Verification items for the finished model (mm, model axes). Round coordinates to 2 decimals unless told otherwise and drop trailing zeros. Order: outer loops, then holes, each group sorted by start corner. A loop starts at its lowest first (then second) coordinate and runs counter-clockwise, first axis right, second up. Notation, with made-up numbers: (45.25, -9.5) -> (66.25, -9.5) arc R32 cw to (66.25, 27.5) -> close; hole circle Ø10 at (18, 26). An arc over 180 degrees is marked (long way). Return JSON: item names as keys, results as strings. Group by question number.
Item 1: Scan lines: probe 1 along Y at (x, z) = (-41, 0.4); probe 2 along X at (y, z) = (-35, 0.4); probe 3 along Y at (x, z) = (-42.25, 0.15). Record each from-to range of solid material in increasing order. Write a range as from..to.
Item 2: Sectioned sample at B-B on x = -40. Record the cut outline in (y, z), plus the area to 3 significant figures.
Item 3: Sectioned sample at A-A on x = -47.25. Record the cut outline in (y, z).
Autodesk Fusion 360 part; units mm, degrees
sketch "Sketch1" plane through (0, 0, 0) normal (0, 0, 1) x (1, 0, 0)
  line L0 (-33, -71.5) -> (-33, -39.0517)
  spline S0 degree 3 poles (-33, -39.0517) (-33, -37.2602) (-33.4854, -35.4836) (-34.2537, -34.2725) (-34.9261, -33.2125) (-35.7722, -32.611) (-36.5563, -32.4575) (-37.1254, -32.346) (-37.6904, -32.44) (-38.2678, -32.7734) knots -1.570796 -1.570796 -1.570796 -1.570796 -0.801145 -0.801145 -0.801145 -0.12753 -0.12753 -0.12753 0.361367 0.361367 0.361367 0.361367
  line L1 (-38.2678, -32.7734) -> (-50, -39.547)
  line L2 (-50, -39.547) -> (-50, -71.5)
  line L3 (-50, -71.5) -> (-33, -71.5)
  line L4 (-33.2, -71.3) -> (-33.2, -39.0517)
  spline S1 degree 3 poles (-33.2, -39.0517) (-33.2, -37.2964) (-33.6813, -35.5482) (-34.4225, -34.3796) (-35.0726, -33.3548) (-35.8807, -32.7936) (-36.5947, -32.6537) (-37.1185, -32.5512) (-37.6252, -32.6333) (-38.1678, -32.9466) knots -1.570796 -1.570796 -1.570796 -1.570796 -0.801145 -0.801145 -0.801145 -0.12753 -0.12753 -0.12753 0.361367 0.361367 0.361367 0.361367
  line L5 (-38.1678, -32.9466) -> (-49.8, -39.6625)
  line L6 (-49.8, -39.6625) -> (-49.8, -71.3)
  line L7 (-49.8, -71.3) -> (-33.2, -71.3)
  dimension "d1" = 17
  dimension "d2" = 71.5
  dimension "d3" = 39.0517
  dimension "d4" = 33
  dimension "d5" = 120
  dimension "d6" = 6.2783
  dimension "d7" = -0.2
extrude "Extrude1" add sketch "Sketch1" along normal blind 0.6 contours L4 S1 L5 L6 L7
Recorded:
{
 "1": {"probe 1": "-71.3..-34.58", "probe 2": "-41.72..-34.08", "probe 3": "-71.3..-35.3"},
 "2": {"outline": "(-71.3, 0) -> (-34, 0) -> (-34, 0.6) -> (-71.3, 0.6) -> close", "area": "22.4 mm²"},
 "3": {"outline": "(-71.3, 0) -> (-38.19, 0) -> (-38.19, 0.6) -> (-71.3, 0.6) -> close"}
}
